from build123d import *

# Parameters (mm, degrees)
SKETCH1_R           = 75
BOSS_EXTRUDE1_DEPTH = 40
SKETCH2_R           = 60
CUT_EXTRUDE1_DEPTH  = 17
SKETCH3_R           = 25
CUT_EXTRUDE2_DEPTH  = 24
SKETCH4_R           = 3
CUT_EXTRUDE3_DEPTH  = 24
SKETCH6_R           = 60
CUT_EXTRUDE4_DEPTH  = 17
SKETCH7_R           = 65
CUT_EXTRUDE5_DEPTH  = 1
SKETCH8_R           = 65
CUT_EXTRUDE6_DEPTH  = 1


with BuildPart() as part:
    # Sketch1 → Boss-Extrude1 (new body)
    with BuildSketch(Plane(origin=(0, 0, 0), x_dir=(1, 0, 0), z_dir=(0, 1, 0))):
        Circle(SKETCH1_R)
    extrude(amount=BOSS_EXTRUDE1_DEPTH)

    # Sketch2 → Cut-Extrude1 (cut)
    with BuildSketch(Plane(origin=(0, 40, 0), x_dir=(1, 0, 0), z_dir=(0, 1, 0))):
        Circle(SKETCH2_R)
    extrude(amount=-CUT_EXTRUDE1_DEPTH, mode=Mode.SUBTRACT)

    # Sketch3 → Cut-Extrude2 (cut, through all)
    with BuildSketch(Plane(origin=(0, 23, 0), x_dir=(1, 0, 0), z_dir=(0, 1, 0))):
        Circle(SKETCH3_R)
    extrude(amount=-CUT_EXTRUDE2_DEPTH, mode=Mode.SUBTRACT)

    # Sketch4 → Cut-Extrude3 (cut, through all)
    with BuildSketch(Plane(origin=(0, 23, 0), x_dir=(1, 0, 0), z_dir=(0, 1, 0))):
        with Locations((0, 35)):
            Circle(SKETCH4_R)
        with Locations((30.310889132, 17.5)):
            Circle(SKETCH4_R)
        with Locations((30.310889132, -17.5)):
            Circle(SKETCH4_R)
        with Locations((0, -35)):
            Circle(SKETCH4_R)
        with Locations((-30.310889132, -17.5)):
            Circle(SKETCH4_R)
        with Locations((-30.310889132, 17.5)):
            Circle(SKETCH4_R)
    extrude(amount=-CUT_EXTRUDE3_DEPTH, mode=Mode.SUBTRACT)

    # Sketch6 → Cut-Extrude4 (cut)
    with BuildSketch(Plane.XZ):
        Circle(SKETCH6_R)
    extrude(amount=-CUT_EXTRUDE4_DEPTH, mode=Mode.SUBTRACT)

    # Sketch7 → Cut-Extrude5 (cut)
    with BuildSketch(Plane.XZ):
        Circle(SKETCH7_R)
    extrude(amount=-CUT_EXTRUDE5_DEPTH, mode=Mode.SUBTRACT)

    # Sketch8 → Cut-Extrude6 (cut)
    with BuildSketch(Plane(origin=(0, 40, 0), x_dir=(1, 0, 0), z_dir=(0, 1, 0))):
        Circle(SKETCH8_R)
    extrude(amount=-CUT_EXTRUDE6_DEPTH, mode=Mode.SUBTRACT)


solid = part.part
Verification items for the finished model (mm, model axes). A direction names the side the tool comes from. Coordinates: 2 decimals unless noted, no trailing zeros. Order: outer loops, then holes, each group sorted by start corner. A loop starts at its lowest first (then second) coordinate and runs counter-clockwise, first axis right, second up.
1. Sectioned sample at B-B, the plane x = 10. Record the cut outline in (y, z).
Results found:
outline: (0, -74.33) - (40, -74.33) - (40, -64.23) - (39, -64.23) - (39, -59.16) - (23, -59.16) - (23, -22.91) - (17, -22.91) - (17, -59.16) - (1, -59.16) - (1, -64.23) - (0, -64.23) - close; (0, 64.23) - (1, 64.23) - (1, 59.16) - (17, 59.16) - (17, 22.91) - (23, 22.91) - (23, 59.16) - (39, 59.16) - (39, 64.23) - (40, 64.23) - (40, 74.33) - (0, 74.33) - close
2. Sectioned sample at A-A, the plane z = 0. Record the cut outline in (x, y).
Results found:
outline: (-75, 0) - (-65, 0) - (-65, 1) - (-60, 1) - (-60, 17) - (-25, 17) - (-25, 23) - (-60, 23) - (-60, 39) - (-65, 39) - (-65, 40) - (-75, 40) - close; (25, 17) - (60, 17) - (60, 1) - (65, 1) - (65, 0) - (75, 0) - (75, 40) - (65, 40) - (65, 39) - (60, 39) - (60, 23) - (25, 23) - close
3. Go/stop test with flat-tipped pins: pin 1 Ø8 at (x, z) = (0, -35) entering from -Y; pin 2 Ø12 at (x, y) = (17.5, 11.5) entering from +Z; pin 3 Ø4 at (x, z) = (39, 6.5) entering from +Y; pin 4 Ø3.5 at (x, z) = (30.31, 17.5) entering from -Y. Record where each tip stops, or that it passes through.
Results found:
pin 1: stops at y = 17
pin 2: stops at z = 74.11
pin 3: stops at y = 23
pin 4: passes through
4. Sectioned sample at C-C, the plane z = 17.5. Give the number of separate pieces and of enclosed holes in the cut face, and give its area (3 significant figures).
Results found:
separate pieces: 4
enclosed holes: 0
area: 1,620 mm2
5. Set-up check for faces 1 (the face through (0, 20, 32)), 2 (the face through (26, 23, -1)), 3 (the face through (-59.94, 8.89, 2.64)): record each of +Z, -Z, +X, -X, +Y, -Y from which the full face is reachable in a straight line by a thin tool's end or side.
Results found:
face 1: +Y, -Y
face 2: +Y
face 3: -Y
6. Release check for a two-part mould opening along X. For faces 4 (the face through (19, 1, -57.5)), 5 (the face through (-9.764, 19.72, -74.362)), 6 (the face through (-23, 0, -61)) record: +X half, -X half, draft (parallel to the pull), parting line (faces both ways), or undercut.
Results found:
face 4: undercut
face 5: parting line
face 6: draft
7. Sectioned sample at D-D, the plane y = 35. Record the cut outline in (x, z), and give its area (3 significant figures).
Results found:
outline: circle Ø150 at (0, 0); hole circle Ø120 at (0, 0)
area: 6,360 mm2
8. Scan lines: line 1 (Z direction, x = 0, y = 20.95); line 2 (Z direction, x = 0, y = 39.7); line 3 (Z direction, x = 0, y = 35). Record each from-to range of solid material in increasing order.
Results found:
line 1: z = -75 to -38, -32 to -25, 25 to 32, 38 to 75
line 2: z = -75 to -65, 65 to 75
line 3: z = -75 to -60, 60 to 75
